Input: dimensioned drawing with shaded views. Units: mm. Origin: part minimum x, y, z. A direction names the side the tool comes from. Coordinates: 2 decimals unless noted, no trailing zeros. Order: outer loops, then holes, each group sorted by start corner. A loop starts at its lowest first (then second) coordinate and runs counter-clockwise, first axis right, second up. Notation, with made-up numbers: (-38.75, 22.5) -> (-17.75, 22.5) arc R13 ccw to (-17.75, 36.5) -> close; hole circle Ø1 at (40.25, -23.5). An arc over 180 degrees is marked (long way). Answer in a Markdown table with one row per item. Add a question column.
1) Contact query for flat-ended pins moving along their axis: P1, Ø6, axis at y = 49, z = 39, coming from the -X side; P2, Ø3, axis at y = 16.5, z = 16.5, coming from the -X side; P3, Ø4.5, axis at x = 8.509, z = 30.48, coming from the -Y side; P4, Ø4, axis at x = 8.5, z = 24, coming from the -Y side. Output: stop coordinate, or through.
2) Section query D-D on y = 52.5. Return the cut outline in (x, z).
3) Set-up query: the marked faces 1, 2, 3 and 4. Return all of +Z, -Z, +X, -X, +Y, -Y with unobstructed straight access to the full face (end or side cutting, diameter ignored); none if empty.
4) Section query A-A on y = 17.5. Return the cut outline in (x, z) (1 decimal).
5) Pull-direction query (X, two-part tool) for the marked faces 5, 6 and 7; classes: +X half, -X half, draft (parallel to the pull), parting line (faces both ways), or undercut.
6) Ray query, line 1 (Y direction, x = 51, z = 40.5); line 2 (X direction, y = 53, z = 30) (1 decimal); line 3 (Z direction, x = 22, y = 32.5). Return the intervals inside material, ascending. Write a range as from..to.
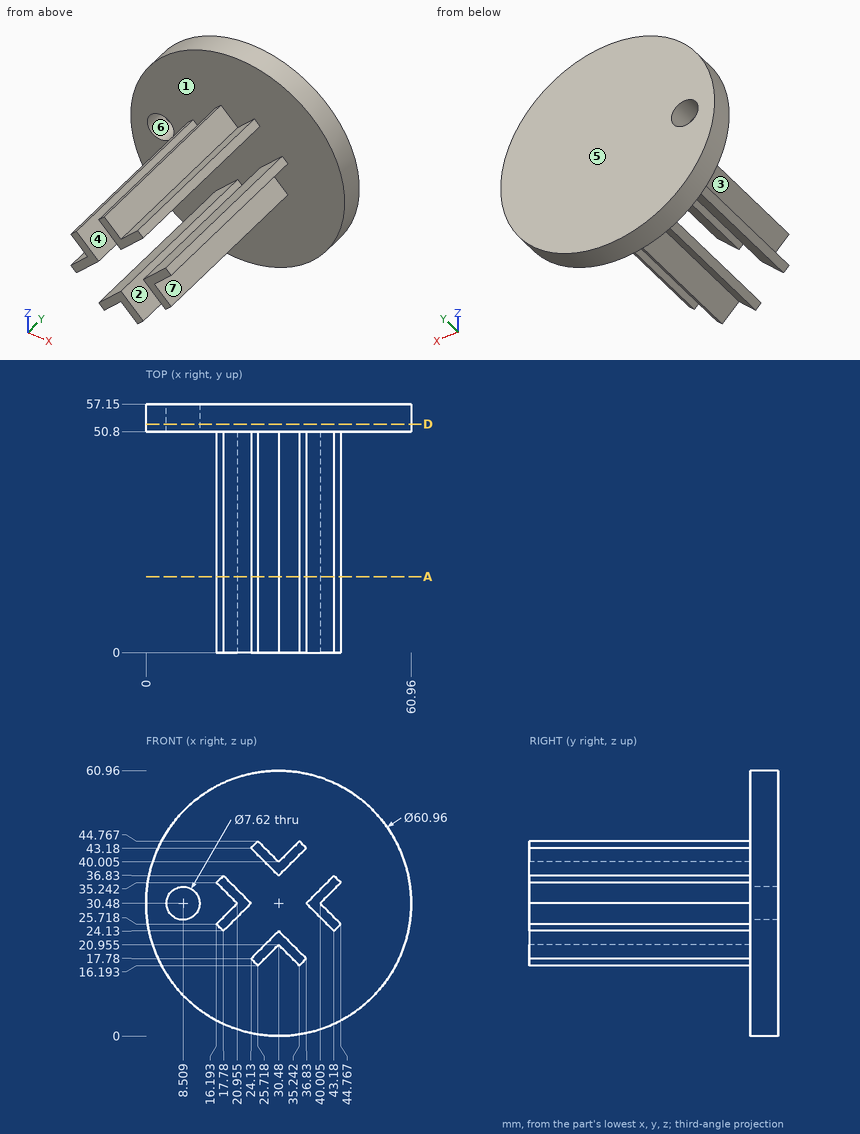
Result:
| question | item | result |
|---|---|---|
| 1 | P1 | x = 0.62 |
| 1 | P2 | x = 24.13 |
| 1 | P3 | through |
| 1 | P4 | y = 50.8 |
| 2 | outline | circle Ø60.96 at (30.48, 30.48); hole circle Ø7.62 at (8.51, 30.48) |
| 3 | face 1 | -Y |
| 3 | face 2 | +X, -Y |
| 3 | face 3 | -X, -Y |
| 3 | face 4 | +Z, -Y |
| 4 | outline | (16.2, 25.7) -> (17.8, 24.1) -> (24.1, 30.5) -> (17.8, 36.8) -> (16.2, 35.2) -> (21, 30.5) -> close; (24.1, 17.8) -> (25.7, 16.2) -> (30.5, 21) -> (35.2, 16.2) -> (36.8, 17.8) -> (30.5, 24.1) -> close; (24.1, 43.2) -> (30.5, 36.8) -> (36.8, 43.2) -> (35.2, 44.8) -> (30.5, 40) -> (25.7, 44.8) -> close; (36.8, 30.5) -> (43.2, 24.1) -> (44.8, 25.7) -> (40, 30.5) -> (44.8, 35.2) -> (43.2, 36.8) -> close |
| 5 | face 5 | draft |
| 5 | face 6 | undercut |
| 5 | face 7 | +X half |
| 6 | line 1 | 50.8..57.15 |
| 6 | line 2 | 0..4.7, 12.3..61 |
| 6 | line 3 | 28.35..32.61 |
